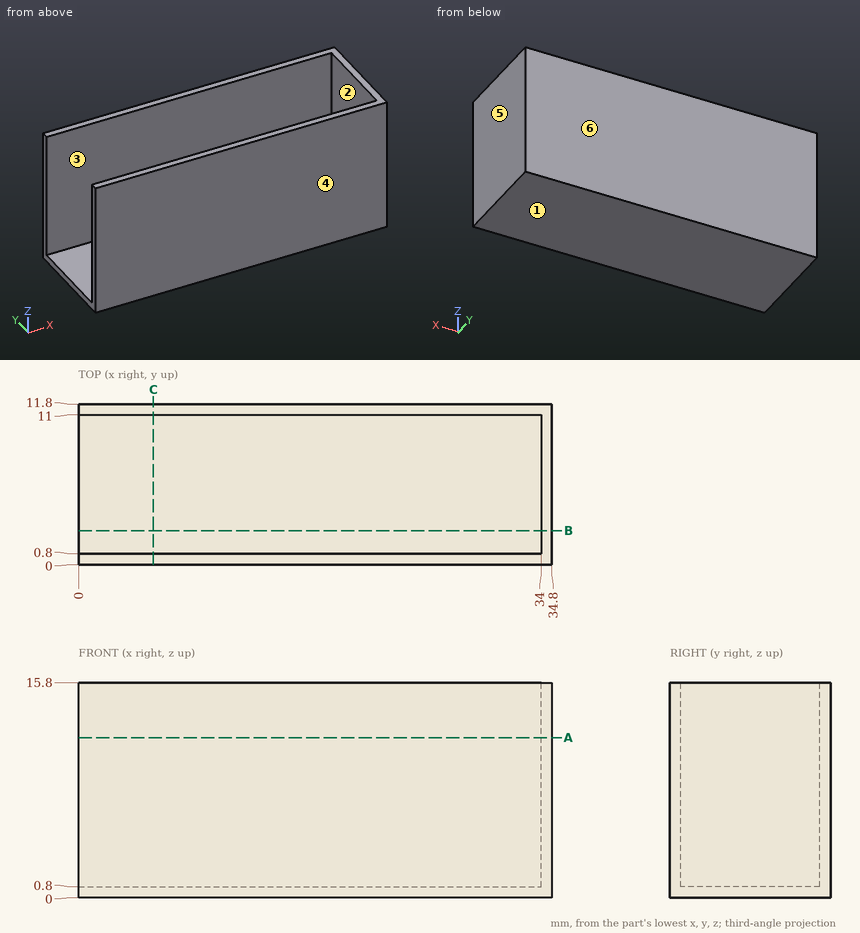
Geometry: see drawing. Coordinates: mm, zero at the bounding-box minimum. A direction names the side the tool comes from. Give positions to 0.01 mm unless a question says otherwise; leave off trailing zeros. Loops run counter-clockwise (first coordinate to the right, second up) from the corner with the lowest first, then second, coordinate; pieces in that order, holes last. Notation, with made-up numbers: M -34.5,58.5 L -3.5,58.5 A24 ccw -3.5,74.5 Z; hole C 42,22 d5. An arc over 180 degrees is marked long. Answer as CSV lines item,"result". Start each with the question number.
1. Reachability of the marked faces 1 and 2 from +Z, -Z, +X, -X, +Y, -Y: full face, straight path, thin tool, end or side. Return the list, or none.
2. Pin query (flat end, axial travel): P1, Ø1.5, axis at y = 10.5, z = 8, coming from the -X side; P2, Ø1, axis at x = 6.5, y = 8.5, coming from the +Z side; P3, Ø1, axis at y = 3, z = 1.5, coming from the -X side. Return the tip coordinate at first contact, or that it passes through.
3. Section C-C on x = 5.5. Return loops of the section in (y, z).
4. Line query: L1, parallel to Y at x = 29.5, z = 14; L2, parallel to X at y = 10.75, z = 6.5; L3, parallel to Z at x = 12.5, y = 5.5. Output: solid intervals per line, ascending.
5. Section A-A on z = 11.75. Return loops of the section in (x, y), plus the area to 3 significant figures.
6. Section B-B on y = 2.5. Return loops of the section in (x, z), plus the area to 3 significant figures.
7. Pull-direction query (Y, two-part tool) for the marked faces 3, 4, 5 and 6; classes: released by +Y, released by -Y, zero draft, split by the parting line, or undercut.
Computed values:
1,face 1,"-Z, +X, -X, +Y, -Y"
1,face 2,"+Z, -X"
2,P1,"stops at x = 0"
2,P2,"stops at z = 0.8"
2,P3,"stops at x = 34"
3,outline,"M 0,0 L 11.8,0 L 11.8,15.8 L 11,15.8 L 11,0.8 L 0.8,0.8 L 0.8,15.8 L 0,15.8 Z"
4,L1,"y = 0 to 0.8, 11 to 11.8"
4,L2,"x = 34 to 34.8"
4,L3,"z = 0 to 0.8"
5,outline,"M 0,0 L 34.8,0 L 34.8,11.8 L 0,11.8 L 0,11 L 34,11 L 34,0.8 L 0,0.8 Z"
5,area,"63.8 mm²"
6,outline,"M 0,0 L 34.8,0 L 34.8,15.8 L 34,15.8 L 34,0.8 L 0,0.8 Z"
6,area,"39.8 mm²"
7,face 3,"undercut"
7,face 4,"released by -Y"
7,face 5,"zero draft"
7,face 6,"released by +Y"
